Autodesk Inventor part; units mm, degrees
ref_plane "Work Plane1" through (29, 0, 0) normal (0, -1, 0) x (1, 0, 0)
ref_plane "YZ Plane" through (0, 0, 0) normal (1, 0, 0) x (0, 1, 0)
ref_plane "XZ Plane" through (0, 0, 0) normal (0, 1, 0) x (-1, 0, 0)
sketch "Sketch1" plane through (0, 0, 0) normal (0, 0, 1) x (1, 0, 0)
  line L0 (-0.8667, 0) -> (6, 0)
  line L1 (6, 0) -> (6, 1.5)
  line L2 (6, 1.5) -> (1.5, 1.5)
  line L3 (1.5, 1.5) -> (1.1932, 1.5)
  line L4 (1.1932, 1.5) -> (0, 1.5)
  line L5 (0, 1.5) -> (0, 2.75)
  line L6 (0, 2.75) -> (-3, 2.75)
  line L7 (-3, 2.75) -> (-3, 1.4434)
  line L8 (-3, 1.4434) -> (-1.7, 1.4434)
  line L9 (-1.7, 1.4434) -> (-0.8667, 0)
  line L10 (-4.8, 0) -> (7.8, 0)
  line L11 (0, -0.55) -> (0, 3.3)
  line L12 (1.5, 1.5) -> (0, 1.5) construction
  dimension "d1" = 4.5
  dimension "d2" = 0.3068
  dimension "d3" = 3
  dimension "d4" = 1.3
  dimension "d5" = 60
  dimension "d6" = 3
  dimension "d7" = 3
  dimension "d8" = 2.8868
  dimension "d9" = 5.5
  dimension "d26" = 6
revolve "Body" add sketch "Sketch1" angle 360 about axis through (-0.8667, 0, 0) along (1, 0, 0)
sketch "Sketch2" plane through (-3, 0, 0) normal (-1, 0, 0) x (0, 0, 1)
  circle A0 centre (0, 0) radius 1.4434
  line L0 (0, -3.85) -> (0, 3.85)
  line L1 (-3.85, 0) -> (3.85, 0)
  line L2 (1.4434, 0) -> (0.7217, -1.25)
  line L3 (0.7217, -1.25) -> (-0.7217, -1.25)
  line L4 (-0.7217, -1.25) -> (-1.4434, 0)
  line L5 (-1.4434, 0) -> (-0.7217, 1.25)
  line L6 (-0.7217, 1.25) -> (0.7217, 1.25)
  line L7 (0.7217, 1.25) -> (1.4434, 0)
  point P0 (0, 0)
extrude "Slot" add sketch "Sketch2" against normal up to next contours L7 A0 | A0 L2 | L6 L0 A0 | A0 L0 L3 | L0 L6 A0 | A0 L3 L0 | L4 A0 | A0 L5
fillet "Fillet1" radius 0.3 1 edges at (-3, -2.75, 0)
thread "Thread"
chamfer "Chamfer1" distance 0.3067 distance2 0.3067 1 edges at (6, -1.5, 0) measured on face at (6, -0.2617, -0.7882)
ref_plane "Work Plane1" through (29, 0, 0) normal (0, -1, 0) x (1, 0, 0)
fillet "Fillet2" radius 0.1 1 edges at (0, -1.5, 0)
equation "\"d1\" = GEL"
equation "\"d3\" = KOH"
equation "\"d4\" = INTI"
equation "\"d6\" = GD"
equation "\"d7\" = BDM"
equation "\"d8\" = 1.1547 * SW"
equation "\"d9\" = KOD"
equation "\"d26\" = NLG"
equation "\"d30\" = R"
equation "\"d17\" = RR"
equation "\"d13\" = GEL"
equation "\"d15\" = -0.5 * SPD + 0.5 * GD"
equation "\"d16\" = GUL"
equation "\"GD\" = 3"
equation "\"NLG\" = 6"
equation "\"GEL\" = 4.5"
equation "\"KOD\" = 5.5"
equation "\"KOH\" = 3"
equation "\"INTI\" = 1.3"
equation "\"GAL\" = 0.61345 * PTC"
equation "\"GUL\" = 0.61345 * PTC"
equation "\"BDM\" = NND"
equation "\"SW\" = 2.5"
equation "\"RR\" = 0.3"
equation "\"SPD\" = NND - 1.2269 * PTC"
equation "\"R\" = 0.1"
equation "\"TOA\" = 30deg"
equation "\"GD1\" = THREADDIA - 1.2269 * PTC"
equation "\"THREADDIA\" = 3"
equation "\"FAWI\" = 45deg"
equation "\"PTC\" = 0.5"
equation "\"NND\" = 3"
equation "\"E0\" = 1.155 * SW"
properties part number "ISO 4762  - M3 x 6" material "Stainless Steel, 440C"
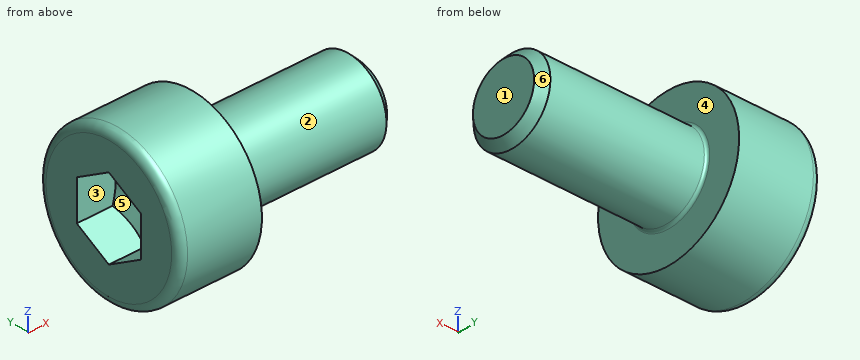
For this review, take the finished solid that the model builds, in its own axes (mm). Face numbers are marked on the shaded views. A direction names the side the tool comes from. Round coordinates to 2 decimals unless told otherwise and drop trailing zeros. Loops run counter-clockwise (first coordinate to the right, second up) from the corner with the lowest first, then second, coordinate; pieces in that order, holes last. Notation, with made-up numbers: (33, 19) - (54, 19) arc R7 ccw to (54, 28) - close; hole circle Ø5 at (-5, 31). An arc over 180 degrees is marked (long way). Answer as CSV lines item,"result".
(1) Insertion check: P1, Ø1.5, axis at x = 3, z = -0.5, coming from the +Y side; P2, Ø2, axis at x = 5, z = 1, coming from the -Y side. Each pin has a flat end and moves straight along its axis. Give the tip position at first contact, or say it passes through.
Checked values:
P1,"stops at y = 1.5"
P2,"stops at y = -1.5"
(2) Consider section C-C on x = -0.25. Give the boundary of the cut face in (y, z).
Checked values:
outline,"circle Ø5.5 at (0, 0)"
(3) Wall thickness on line 1 (X direction, y = 1.6, z = 1.9); line 2 (X direction, y = 0.4, z = -0.2); line 3 (Y direction, x = -1.5, z = 0.35): over which ranges is each line inside the solid? List them lowest first.
Checked values:
line 1,"x = -3 to 0"
line 2,"x = -1.12 to 6"
line 3,"y = -2.73 to -1.04, 1.04 to 2.73"
(4) Consider section B-B on x = -1.25. Give the boundary of the cut face in (y, z), then the cut area to 3 significant figures.
Checked values:
outline,"circle Ø5.5 at (0, 0); hole circle Ø1.33 at (0, 0)"
area,"22.4 mm2"
(5) Mouldability with a two-part tool opening along Y and no side actions: class the marked faces 4, 5 and 6 as +Y half, -Y half, draft (parallel to the pull), parting line (faces both ways), or undercut.
Checked values:
face 4,"draft"
face 5,"undercut"
face 6,"parting line"
(6) Consider section A-A on x = 2. Give the boundary of the cut face in (y, z), then the cut area to 3 significant figures.
Checked values:
outline,"circle Ø3 at (0, 0)"
area,"7.07 mm2"
(7) Tool access review of the marked faces 1, 2 and 3: name each direction out of +Z, -Z, +X, -X, +Y, -Y from which nothing blocks a thin tool from reaching the whole face with its end or side.
Checked values:
face 1,"+Z, -Z, +X, +Y, -Y"
face 2,"+X"
face 3,"-X"
